from build123d import *

# Parameters (mm, degrees)
F0_W     = 80.548994
F0_H     = 65.119892
F1_DEPTH = 50.8
F2_W     = 74.689142
F2_H     = 59.31776
F3_DEPTH = 47.752
F4_R     = 7.108362
F4_R_2   = 5.812962
F5_DEPTH = 2.032


with BuildPart() as f1:
    # F0 (on Top) → F1 (new body)
    with BuildSketch(Plane.XY):
        Rectangle(F0_W, F0_H)
    extrude(amount=F1_DEPTH)

    # F2 (on face) → F3 (cut)
    with BuildSketch(Plane.XY.offset(50.8)):
        Rectangle(F2_W, F2_H)
    extrude(amount=-F3_DEPTH, mode=Mode.SUBTRACT)

    # F4 (on face) → F5 (join)
    with BuildSketch(Plane.XZ.offset(32.559946)):
        with Locations((1.574243, 38.920175)):
            Circle(F4_R)
        with Locations((1.574243, 38.920175)):
            Circle(F4_R_2, mode=Mode.SUBTRACT)
    extrude(amount=F5_DEPTH)


solid = f1.part
Can you work these out from the model? Positions are in its coordinate system, mm. A direction names the side the tool comes from. Give positions to 0.01 mm unless a question says otherwise; leave off trailing zeros. Loops run counter-clockwise (first coordinate to the right, second up) from the corner with the lowest first, then second, coordinate; pieces in that order, holes last. Notation, with made-up numbers: (-26, -23) - (-8, -23) arc R21 cw to (-8, 2) - close; hole circle Ø9 at (5, 56.25). An arc over 180 degrees is marked (long way). Answer as a JSON object with one key per item and string values.
Q1. Will these pins go through, and if not, where does the flat tip stop? P1, Ø4, axis at x = 16.5, y = -26.5, coming from the +Z side; P2, Ø3.5, axis at x = 2, z = 37, coming from the -Y side.
Geometry says:
{"P1": "z = 3.05", "P2": "y = -32.56"}
Q2. Imagine slicing it at A-A on z = 6. Write out the boundary of the cut face in (x, y).
Geometry says:
{"outline": "(-40.27, -32.56) - (40.27, -32.56) - (40.27, 32.56) - (-40.27, 32.56) - close; hole (-37.34, -29.66) - (37.34, -29.66) - (37.34, 29.66) - (-37.34, 29.66) - close"}
Q3. Imagine slicing it at D-D on z = 41. Write out the boundary of the cut face in (x, y).
Geometry says:
{"outline": "(-40.27, -32.56) - (-5.22, -32.56) - (-5.22, -34.59) - (-3.85, -34.59) - (-3.85, -32.56) - (7, -32.56) - (7, -34.59) - (8.37, -34.59) - (8.37, -32.56) - (40.27, -32.56) - (40.27, 32.56) - (-40.27, 32.56) - close; hole (-37.34, -29.66) - (37.34, -29.66) - (37.34, 29.66) - (-37.34, 29.66) - close"}
Q4. Which directions (+Z, -Z, +X, -X, +Y, -Y) give clear straight access to the entire face, cutting with the end or side of a thin tool? Please do faces 5 (the flat face through (-1, 29.659, 27)), 6 (the cylindrical face through (0.65, -33.56, 45.97)), 7 (the flat face through (3, -34.592, 33)).
Geometry says:
{"face 5": "+Z", "face 6": "-Y", "face 7": "+Z, -Z, +X, -X, -Y"}
Q5. If we mould it in two halves opening along Z, with no side actions, what happens to faces 1 (the flat face through (37.345, 0, 27)), 2 (the flat face through (1, -32.56, 39)), 3 (the cylindrical face through (4.257, -33.562, 33.763)), 4 (the flat face through (-1, 0, 3.048))? For each: pulls with the +Z half, pulls with the -Z half, needs draft (parallel to the pull), parting line crosses it, or undercut.
Geometry says:
{"face 1": "needs draft", "face 2": "undercut", "face 3": "undercut", "face 4": "pulls with the +Z half"}
Q6. If I drill on L1, parallel to X at y = 28, z = 16.5; L2, parallel to Y at x = -35, z = 47; L3, parallel to Z at x = 5, y = 29.5, over which ranges is the centre line in solid material (lowest first)?
Geometry says:
{"L1": "-40.27 to -37.34, 37.34 to 40.27", "L2": "-32.56 to -29.66, 29.66 to 32.56", "L3": "0 to 3.05"}
Q7. Imagine slicing it at B-B on x = 35.5. Write out the boundary of the cut face in (y, z), plus the area to 3 significant figures.
Geometry says:
{"outline": "(-32.56, 0) - (32.56, 0) - (32.56, 50.8) - (29.66, 50.8) - (29.66, 3.05) - (-29.66, 3.05) - (-29.66, 50.8) - (-32.56, 50.8) - close", "area": "476 mm²"}
Q8. Imagine slicing it at C-C on y = 2. Write out the boundary of the cut face in (x, z).
Geometry says:
{"outline": "(-40.27, 0) - (40.27, 0) - (40.27, 50.8) - (37.34, 50.8) - (37.34, 3.05) - (-37.34, 3.05) - (-37.34, 50.8) - (-40.27, 50.8) - close"}
